```python
from build123d import *

# Parameters (mm, degrees)
SKETCH1_R           = 17
SKETCH1_R_2         = 2.1
SKETCH1_R_3         = 1.7
BOSS_EXTRUDE1_DEPTH = 4
BOSS_EXTRUDE2_START = -6
SKETCH2_R           = 2.1
BOSS_EXTRUDE2_DEPTH = 6
CUT_EXTRUDE1_START  = -2
SKETCH3_R           = 3
SKETCH3_R_2         = 1.7
CUT_EXTRUDE1_DEPTH  = 2


with BuildPart() as part:
    # Sketch1 → Boss-Extrude1 (new body)
    with BuildSketch(Plane(origin=(0, 292.043042306, 5.097630265), x_dir=(1, 0, 0), z_dir=(0, 0.9998476951563913, 0.017452406437283286))):
        with Locations(Location((109.84658574, -203.196308074, 0), (0, 0, 270))):
            Circle(SKETCH1_R)
        with Locations(Location((120.910918653, -196.961684011, 0), (0, 0, 270))):
            Circle(SKETCH1_R_2, mode=Mode.SUBTRACT)
        with Locations(Location((98.782252828, -209.430932137, 0), (0, 0, 270))):
            Circle(SKETCH1_R_2, mode=Mode.SUBTRACT)
        with Locations(Location((116.081209803, -214.260640986, 0), (0, 0, 270))):
            Circle(SKETCH1_R_3, mode=Mode.SUBTRACT)
        with Locations(Location((103.611961678, -192.131975161, 0), (0, 0, 270))):
            Circle(SKETCH1_R_3, mode=Mode.SUBTRACT)
    extrude(amount=BOSS_EXTRUDE1_DEPTH)

    # Sketch2 → Boss-Extrude2 (add)
    with BuildSketch(Plane(origin=(0, 296.042433086, 5.167439891), x_dir=(1, 0, 0), z_dir=(0, 0.9998476951563913, 0.01745240643728325)).offset(BOSS_EXTRUDE2_START)):
        with Locations(Location((98.782252828, -209.430932137, 0), (0, 0, 270))):
            Circle(SKETCH2_R)
        with Locations(Location((120.910918653, -196.961684011, 0), (0, 0, 270))):
            Circle(SKETCH2_R)
    extrude(amount=BOSS_EXTRUDE2_DEPTH)

    # Sketch3 → Cut-Extrude1 (cut)
    # profile 1 of 2: a face of its own
    with BuildSketch(Plane(origin=(0, 296.042433086, 5.167439891), x_dir=(1, 0, 0), z_dir=(0, 0.9998476951563913, 0.01745240643728325)).offset(CUT_EXTRUDE1_START)):
        with Locations(Location((103.611961678, -192.131975161, 0), (0, 0, 270))):
            Circle(SKETCH3_R)
        with Locations(Location((103.611961678, -192.131975161, 0), (0, 0, 270))):
            Circle(SKETCH3_R_2, mode=Mode.SUBTRACT)
    # profile 2 of 2: a face of its own
    with BuildSketch(Plane(origin=(0, 296.042433086, 5.167439891), x_dir=(1, 0, 0), z_dir=(0, 0.9998476951563913, 0.01745240643728325)).offset(CUT_EXTRUDE1_START)):
        with Locations(Location((116.081209803, -214.260640986, 0), (0, 0, 270))):
            Circle(SKETCH3_R)
        with Locations(Location((116.081209803, -214.260640986, 0), (0, 0, 270))):
            Circle(SKETCH3_R_2, mode=Mode.SUBTRACT)
    extrude(amount=CUT_EXTRUDE1_DEPTH, mode=Mode.SUBTRACT)


solid = part.part
```
Work out the finished part from the listing and answer in its coordinate system (mm). Give positions to 0.01 mm unless a question says otherwise; leave off trailing zeros. Order: outer loops, then holes, each group sorted by start corner. A loop starts at its lowest first (then second) coordinate and runs counter-clockwise, first axis right, second up.
1. The mould has two halves that part along X. Classify faces 1 (the cylindrical face through (113.15, 291.3, 218.73)), 2 (the cylindrical face through (104.513, 291.625, 200.113)), 3 (the cylindrical face through (100.864, 287.379, 214.206)): released by +X, released by -X, zero draft, split by the parting line, or undercut.
Result sheet:
face 1: undercut
face 2: undercut
face 3: split by the parting line
2. Straight lines are drawn through the part: L1, parallel to X at y = 288.75, z = 219.5; L2, parallel to Z at x = 113.5, y = 291; L3, parallel to X at y = 290.25, z = 198. For each, find the intervals that lie inside material, in ascending order.
Result sheet:
L1: x = 97.08 to 114.39, 117.77 to 122.61
L2: z = 191.7 to 217.84, 220.9 to 224.91
L3: x = 96.32 to 102.1, 105.13 to 123.38
3. Each of these flat-tipped pins is pushed along its axis until it touches: P1, Ø3, axis at x = 109.5, z = 195, coming from the -Y side; P2, Ø2, axis at y = 288.5, z = 215.5, coming from the +X side; P3, Ø1, axis at x = 116, z = 203, coming from the +Y side. Where does it stop, or does it pass through?
Result sheet:
P1: stops at y = 288.7
P2: stops at x = 125.66
P3: stops at y = 292.6
4. Section A-A, the plane x = 103 is taken. Determine the outline of the cut face in (y, z).
Result sheet:
outline: (288.23, 223.82) - (288.66, 198.79) - (290.66, 198.82) - (290.64, 200.17) - (292.64, 200.21) - (292.22, 223.89) - close; (288.72, 195.61) - (288.77, 192.71) - (292.77, 192.77) - (292.74, 194.33) - (290.74, 194.3) - (290.72, 195.65) - close
5. Section D-D, the plane x = 107.5 is taken. Determine the outline of the cut face in (y, z), and give its area (3 significant figures).
Result sheet:
outline: (288.2, 225.1) - (288.79, 191.43) - (292.79, 191.5) - (292.2, 225.17) - close
area: 135 mm2
6. Section C-C, the plane y = 291.75 is taken. Give the number of separate pieces and of enclosed holes in the cut face, and give its area (4 significant figures).
Result sheet:
separate pieces: 1
enclosed holes: 2
area: 851.5 mm2
7. Section B-B, the plane x = 124 is taken. Determine the outline of the cut face in (y, z), and give its area (3 significant figures).
Result sheet:
outline: (288.33, 217.68) - (288.66, 198.85) - (292.66, 198.92) - (292.33, 217.75) - close
area: 75.3 mm2
